Source: CAD feature listing. Evaluate the final solid. Frame: model axes, mm. Coordinates: 2 decimals unless noted, no trailing zeros. Order: outer loops, then holes, each group sorted by start corner. A loop starts at its lowest first (then second) coordinate and runs counter-clockwise, first axis right, second up.
Autodesk Inventor part; units mm, degrees
ref_plane "YZ Plane" through (0, 0, 0) normal (1, 0, 0) x (0, 1, 0)
ref_plane "XZ Plane" through (0, 0, 0) normal (0, 1, 0) x (-1, 0, 0)
ref_plane "XY Plane" through (0, 0, 0) normal (0, 0, 1) x (1, 0, 0)
sketch "Sketch1" plane through (0, 0, 0) normal (0, 0, 1) x (1, 0, 0)
  line L0 (-30, 0) -> (30, 0)
  line L1 (30, 0) -> (30, 106)
  line L2 (30, 106) -> (-30, 106)
  line L3 (-30, 106) -> (-30, 0)
  point P0 (0, 0)
  dimension "d0" = 60
  dimension "d1" = 106
  dimension "d2" = 30
extrude "Extrusion1" add sketch "Sketch1" along normal blind 8
fillet "Fillet1" radius 10 2 edges at (30, 106, 4) (-30, 106, 4)
sketch "Sketch2" plane through (0, 0, 8) normal (0, 0, 1) x (1, 0, 0)
  circle A0 centre (0, 72) radius 18
  line L0 (0, 72) -> (-15.5885, 63)
  line L1 (0, 72) -> (0, 90)
  line L2 (0, 72) -> (15.5885, 63)
  point P0 (0, 0)
  point P1 (0, 90)
  point P2 (-15.5885, 63)
  point P3 (15.5885, 63)
  dimension "d6" = 36
  dimension "d7" = 120
  dimension "d8" = 120
  dimension "d9" = 0
  dimension "d10" = 72
hole "Hole1" at (0, 90, 8) at (-15.5885, 63, 8) at (15.5885, 63, 8) direction (0, 0, -1) diameter 6 end through all
sketch "Sketch3" plane through (0, 0, 8) normal (0, 0, 1) x (1, 0, 0)
  circle A0 centre (0, 72) radius 12.5
  line L0 (-30, 0) -> (30, 0)
  point P0 (0, 0)
  dimension "d18" = 72
  dimension "d19" = 0
  dimension "d20" = 25
extrude "Extrusion2" cut sketch "Sketch3" against normal through all
chamfer "Chamfer1" distance 2 angle 45 10 edges at (0, 106, 8) (-27.0711, 103.0711, 8) (-30, 48, 8) (27.0711, 103.0711, 8) (30, 48, 8) (0, 106, 0) (-27.0711, 103.0711, 0) (-30, 48, 0) (27.0711, 103.0711, 0) (30, 48, 0)
equation "\"d18\" = centreHeight + heightClearance"
equation "\"centreHeight\" = 66"
equation "\"heightClearance\" = 6"
properties part number "motorHolder_rotor" material "Steel, Mild"
1. Section query C-C on y = 45. Return loops of the section in (x, z), plus the area to 3 significant figures.
Findings:
outline: (-30, 2) - (-28, 0) - (28, 0) - (30, 2) - (30, 6) - (28, 8) - (-28, 8) - (-30, 6) - close
area: 472 mm2
2. Ray query, line 1 (Y direction, x = 0, z = 2.5); line 2 (X direction, y = 63, z = 2.5); line 3 (X direction, y = 63, z = 6.25). Return the intervals inside material, ascending.
Findings:
line 1: y = 0 to 59.5, 84.5 to 87, 93 to 106
line 2: x = -30 to -18.59, -12.59 to -8.67, 8.67 to 12.59, 18.59 to 30
line 3: x = -29.75 to -18.59, -12.59 to -8.67, 8.67 to 12.59, 18.59 to 29.75
3. Section query D-D on z = 1. Return loops of the section in (x, y).
Findings:
outline: (-29, 0) - (29, 0) - (29, 96) arc R9 ccw to (20, 105) - (-20, 105) arc R9 ccw to (-29, 96) - close; hole circle Ø6 at (-15.59, 63); hole circle Ø25 at (0, 72); hole circle Ø6 at (0, 90); hole circle Ø6 at (15.59, 63)
4. Section query A-A on y = 79.5. Return loops of the section in (x, z).
Findings:
outline: (-30, 2) - (-28, 0) - (-10, 0) - (-10, 8) - (-28, 8) - (-30, 6) - close; (10, 0) - (28, 0) - (30, 2) - (30, 6) - (28, 8) - (10, 8) - close
5. Section query B-B on x = 0. Return loops of the section in (y, z).
Findings:
outline: (0, 0) - (59.5, 0) - (59.5, 8) - (0, 8) - close; (84.5, 0) - (87, 0) - (87, 8) - (84.5, 8) - close; (93, 0) - (104, 0) - (106, 2) - (106, 6) - (104, 8) - (93, 8) - close
6. Draft query along Y for faces 1 (the face through (0, 93, 4)), 2 (the face through (0, 53, 8)), 3 (the face through (0, 0, 4)). Return one class per face: released by +Y, released by -Y, zero draft, split by the parting line, or undercut.
Findings:
face 1: undercut
face 2: zero draft
face 3: released by -Y
